```python
from build123d import *

# Parameters (mm, degrees)
SKETCH1_W           = 90
SKETCH1_H           = 40
BOSS_EXTRUDE1_DEPTH = 2
SKETCH4_R           = 2
BOSS_EXTRUDE2_DEPTH = 80


with BuildPart() as part:
    # Sketch1 → Boss-Extrude1 (new, symmetric)
    with BuildSketch(Plane.XY):
        with Locations((45, 0)):
            Rectangle(SKETCH1_W, SKETCH1_H)
    extrude(amount=BOSS_EXTRUDE1_DEPTH, both=True)

    # Sketch4 → Boss-Extrude2 (add)
    with BuildSketch(Plane.XZ.offset(20)):
        with Locations(Location((0, 0, 0), (0, 0, 270))):
            Circle(SKETCH4_R)
    extrude(amount=-BOSS_EXTRUDE2_DEPTH)


solid = part.part
```
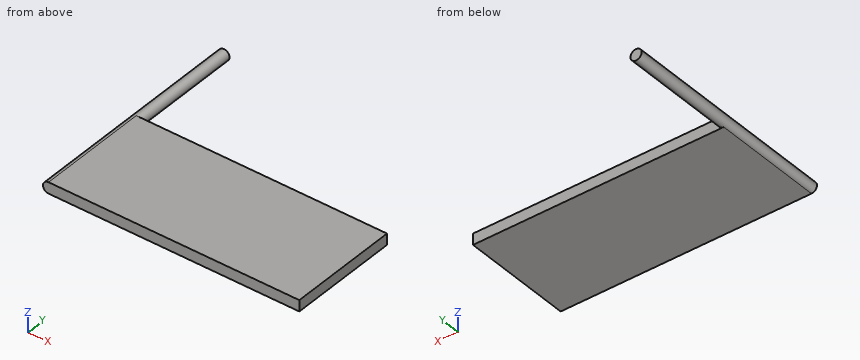
Part model, mm, in its own coordinate system. Give positions to 0.01 mm unless a question says otherwise; leave off trailing zeros. Order: outer loops, then holes, each group sorted by start corner. A loop starts at its lowest first (then second) coordinate and runs counter-clockwise, first axis right, second up. Notation, with made-up numbers: M 0,-30 L 55,-30 A18 cw 55,-9 Z; hole C -8.5,86 d8. An arc over 180 degrees is marked long. Use a Markdown table: item, result. Add a question column.
(1) Saw through at B-B, the plane x = 25. Give the cut face in (y, z), and give its area (3 significant figures).
(2) Probe line 1 along Y through (x, z) = (40.5, -0.35); line 2 along X through (y, z) = (-3, 0.15); line 3 along X through (y, z) = (44.5, -0.15). List the from-to ranges inside material, lowest first. Write a range as [from, to].
(3) Drop flat-ended pins along their axis: P1, Ø1, axis at y = 42, z = -1, coming from the -X side; P2, Ø1.5, axis at x = 11.5, z = 1, coming from the +Y side. Give the stop position or say it passes through.
(4) Saw through at A-A, the plane z = 0. Give the cut face in (x, y), and give its area (3 significant figures).
(5) Saw through at C-C, the plane y = 39.5. Give the cut face in (x, z).
Answer key:
| question | item | result |
|---|---|---|
| 1 | outline | M -20,-2 L 20,-2 L 20,2 L -20,2 Z |
| 1 | area | 160 mm^2 |
| 2 | line 1 | [-20, 20] |
| 2 | line 2 | [-1.99, 90] |
| 2 | line 3 | [-1.99, 1.99] |
| 3 | P1 | x = -1.94 |
| 3 | P2 | y = 20 |
| 4 | outline | M -2,-20 L 90,-20 L 90,20 L 2,20 L 2,60 L -2,60 Z |
| 4 | area | 3,840 mm^2 |
| 5 | outline | C 0,0 d4 |
